```python
from build123d import *

# Parameters (mm, degrees)
SKETCH1_R           = 11
BOSS_EXTRUDE1_DEPTH = 46
SKETCH2_R           = 7.5
BOSS_EXTRUDE2_DEPTH = 18
SKETCH3_R           = 7.5
BOSS_EXTRUDE3_DEPTH = 18


with BuildPart() as part:
    # Sketch1 → Boss-Extrude1 (new body)
    with BuildSketch(Plane(origin=(0, 0, 0), x_dir=(0, 0, -1), z_dir=(1, 0, 0))):
        Circle(SKETCH1_R)
    extrude(amount=BOSS_EXTRUDE1_DEPTH)

    # Sketch2 → Boss-Extrude2 (add)
    with BuildSketch(Plane(origin=(46, 0, 0), x_dir=(0, 0, -1), z_dir=(1, 0, 0))):
        Circle(SKETCH2_R)
    extrude(amount=BOSS_EXTRUDE2_DEPTH)

    # Sketch3 → Boss-Extrude3 (add)
    with BuildSketch(Plane.ZY):
        Circle(SKETCH3_R)
    extrude(amount=BOSS_EXTRUDE3_DEPTH)


solid = part.part
```
Design review of the part built by this model. Coordinates are the model's own, in mm. A direction names the side the tool comes from. Give positions to 0.01 mm unless a question says otherwise; leave off trailing zeros. Order: outer loops, then holes, each group sorted by start corner. A loop starts at its lowest first (then second) coordinate and runs counter-clockwise, first axis right, second up. Notation, with made-up numbers: (14, 67.5) -> (42, 67.5) arc R18 cw to (42, 75.5) -> close; hole circle Ø4 at (39.5, -27). An arc over 180 degrees is marked (long way). Write each question's results on one line, items separated by ' | '. Start each with the question number.
Q1. Add section A-A on y = 0. Give the boundary of the cut face in (x, z), and give its area (3 significant figures).
Q2. Machinability: for faces 1 (the flat face through (46, 2.6, -7.2)), 2 (the flat face through (64, 0, 0)), 3 (the cylindrical face through (-8.874, 0.33, -7.493)), which of the approach directions +Z, -Z, +X, -X, +Y, -Y give a long, thin tool a straight path to every point of the face, cutting with its end or side? Answer none if there is none.
Q3. Add section C-C on x = 55. Give the boundary of the cut face in (y, z), and give its area (3 significant figures).
Q4. Wall thickness on L1, parallel to X at y = 8.75, z = 6.5; L2, parallel to Y at x = 40.5, z = -0.5; L3, parallel to Y at x = -10, z = -5.75: over which ranges is each line inside the solid? List them lowest first. Write a range as from..to.
Q5. For pin 1 (1 mm diameter, centred on y = -5.5, z = 8, fed in from -X); pin 2 (4 mm diameter, centred on x = 40.5, y = -5.5, fed in from -Z); pin 3 (1 mm diameter, centred on x = 28.5, z = -7.5, fed in from -Y), all flat-tipped, find the tip position at first contact; note any pin that passes through.
Q6. Add section D-D on x = 36. Give the boundary of the cut face in (y, z).
Found:
1) outline: (-18, -7.5) -> (0, -7.5) -> (0, -11) -> (46, -11) -> (46, -7.5) -> (64, -7.5) -> (64, 7.5) -> (46, 7.5) -> (46, 11) -> (0, 11) -> (0, 7.5) -> (-18, 7.5) -> close | area: 1,550 mm2
2) face 1: +X | face 2: +Z, -Z, +X, +Y, -Y | face 3: -X
3) outline: circle Ø15 at (0, 0) | area: 177 mm2
4) L1: x = 0..46 | L2: y = -10.99..10.99 | L3: y = -4.82..4.82
5) pin 1: stops at x = 0 | pin 2: stops at z = -10.43 | pin 3: stops at y = -8.49
6) outline: circle Ø22 at (0, 0)
